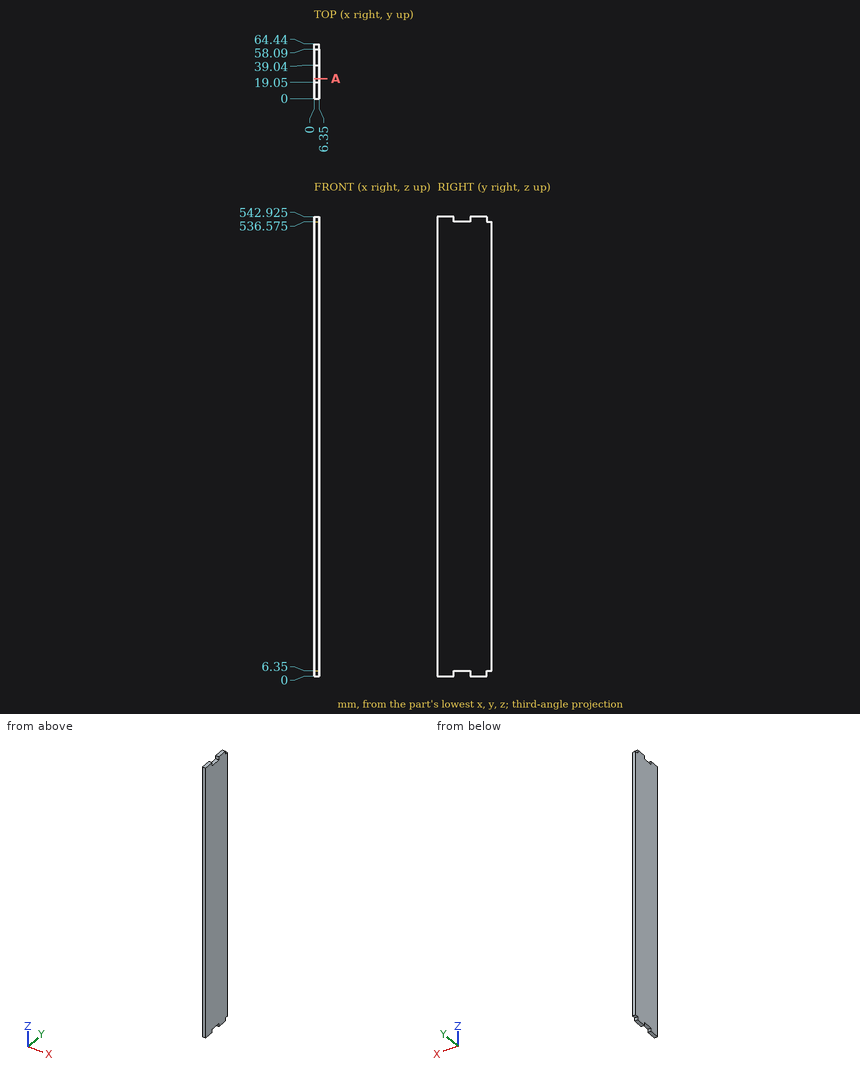
Could you check a few things on this drawing? It's one solid part, dimensions in mm from its lowest x, y, z. Give positions to 0.01 mm unless a question says otherwise; leave off trailing zeros. Write each loop counter-clockwise with the first axis right and the second up, starting at its lowest first coordinate (ties: lowest second). Pieces come first, ordered by that corner, then holes. Notation, with made-up numbers: M -2.75,42.25 L 1.25,42.25 A14 cw 1.25,68.25 Z; hole C 0.5,51.5 d4. An arc over 180 degrees is marked long. Put each result on its own line as item: value. Start each with the question number.
Item 1: I need wall thicknesses on L1, parallel to Z at x = 3.75, y = 22.5 (3 decimals). Which ranges of the line are inside material? Lowest first, please. Write a range as from..to.
Item 2: Will these pins go through, and if not, where does the flat tip stop? pin 1 (1.9 mm diameter, centred on x = 3, y = 34, fed in from -Z); pin 2 (1.9 mm diameter, centred on x = 2.5, y = 60, fed in from +Z) (3 decimals); pin 3 (1.9 mm diameter, centred on x = 2.5, z = 539.5, fed in from +Y).
Item 3: If we section it at A-A, the plane y = 23.5: Write out the boundary of the cut face in (x, z) (3 decimals).
Values:
1. L1: 6.35..536.575
2. pin 1: z = 6.35
2. pin 2: z = 536.575
2. pin 3: y = 58.09
3. outline: M 0,6.35 L 6.35,6.35 L 6.35,536.575 L 0,536.575 Z
